from build123d import *

# Parameters (mm, degrees)
T_LE_DE_BASE_PLI_E1_DEPTH = 20
ESQUISSE7_R               = 2
ENL_V_MAT_EXTRU_1_DEPTH   = 25.586228611
ENL_V_MAT_EXTRU_2_DEPTH   = 25.586228611


# Sheet-metal steps are written as plain solids
with BuildPart() as part:
    # Esquisse2 → Tôle de base pliée1 (new body)
    with BuildSketch(Plane.XY):
        with BuildLine():
            Line((-8.571428571, 10.221674877), (-8.571428571, -2.778325123))
            ThreePointArc((-8.571428571, -2.778325123), (-7.985642134, -4.192538686), (-6.571428571, -4.778325123))
            Line((-6.571428571, -4.778325123), (-0.571428571, -4.778325123))
            ThreePointArc((-0.571428571, -4.778325123), (0.842784991, -4.192538686), (1.428571429, -2.778325123))
            Line((1.428571429, -2.778325123), (1.428571429, 10.221674877))
            Line((1.428571429, 10.221674877), (0.428571429, 10.221674877))
            Line((0.428571429, 10.221674877), (0.428571429, -2.778325123))
            ThreePointArc((0.428571429, -2.778325123), (0.13567821, -3.485431904), (-0.571428571, -3.778325123))
            Line((-0.571428571, -3.778325123), (-6.571428571, -3.778325123))
            ThreePointArc((-6.571428571, -3.778325123), (-7.278535353, -3.485431904), (-7.571428571, -2.778325123))
            Line((-7.571428571, -2.778325123), (-7.571428571, 10.221674877))
            Line((-7.571428571, 10.221674877), (-8.571428571, 10.221674877))
        make_face()
    extrude(amount=T_LE_DE_BASE_PLI_E1_DEPTH)

    # Esquisse7 → Enlèv. mat.-Extru.1 (cut, through all)
    with BuildSketch(Plane(origin=(1.428571429, 0, 0), x_dir=(0, 0, -1), z_dir=(1, 0, 0))):
        with Locations(Location((-3, 7.221674877, 0), (0, 0, 180))):
            Circle(ESQUISSE7_R)
        with Locations((-17, 0.221674877)):
            Circle(ESQUISSE7_R)
        with BuildLine():
            Line((-18.341640786, 2.90495645), (-4.341640786, 9.90495645))
            ThreePointArc((-4.341640786, 9.90495645), (-3.689258762, 10.141421845), (-3, 10.221674877))
            Line((-3, 10.221674877), (-20, 10.221674877))
            Line((-20, 10.221674877), (-20, 0.221674877))
            ThreePointArc((-20, 0.221674877), (-19.551952425, 1.798868213), (-18.341640786, 2.90495645))
        make_face()
    extrude(amount=-ENL_V_MAT_EXTRU_1_DEPTH, mode=Mode.SUBTRACT)

    # Esquisse9 → Enlèv. mat.-Extru.2 (cut, through all)
    with BuildSketch(Plane(origin=(1.428571429, 0, 0), x_dir=(0, 0, -1), z_dir=(1, 0, 0))):
        with BuildLine():
            Line((-3, 10.221674877), (0, 10.221674877))
            Line((0, 10.221674877), (0, 7.221674877))
            ThreePointArc((0, 7.221674877), (-0.878679656, 9.34299522), (-3, 10.221674877))
        make_face()
    extrude(amount=-ENL_V_MAT_EXTRU_2_DEPTH, mode=Mode.SUBTRACT)


solid = part.part
Could you check a few things on this model? Use its own coordinates, in mm. A direction names the side the tool comes from. Give positions to 0.01 mm unless a question says otherwise; leave off trailing zeros. Loops run counter-clockwise (first coordinate to the right, second up) from the corner with the lowest first, then second, coordinate; pieces in that order, holes last. Notation, with made-up numbers: (49.5, 46) -> (85.5, 46) arc R24 cw to (85.5, 85) -> close; hole circle Ø7 at (30.5, 85.5). An arc over 180 degrees is marked (long way). Answer as CSV lines item,"result". Start each with the question number.
(1) I'm going to push flat-ended pins straight in: pin 1 Ø1.5 at (x, z) = (0, 12.5) entering from +Y; pin 2 Ø5 at (x, z) = (-2.5, 9.5) entering from +Y; pin 3 Ø4 at (x, z) = (-5, 12.5) entering from +Y. Where does each tip first touch, or does it pass through?
(2) If we section it at A-A on y = 1: Write out the boundary of the cut face in (x, z).
(3) I need wall thicknesses on probe 1 along X at (y, z) = (1.75, 10.25); probe 2 along Y at (x, z) = (-3, 4.5); probe 3 along Y at (x, z) = (-8.05, 17). Which ranges of each line are inside material? Lowest first, please.
(4) Which directions (+Z, -Z, +X, -X, +Y, -Y) give clear straight access to the entire face, cutting with the end or side of a thin tool? Please do faces 1 (the cylindrical face through (-7.271, -3.493, 9.86)), 2 (the cylindrical face through (-8.1, 0.3, 19)).
(5) If we section it at B-B on z = 3.5: Write out the boundary of the cut face in (x, y), then the cut area to 3 significant figures.
(6) If we section it at D-D on y = 9.5: Write out the boundary of the cut face in (x, z).
(7) We'd pull the mould along X, two halves only. Please class faces 3 (the flat face through (-8.571, 2, 8)), 4 (the flat face through (0.429, 2, 8)), 5 (the flat face through (-4, -4.778, 10)): released by +X, released by -X, zero draft, split by the parting line, or undercut.
(8) If we section it at C-C on x = 0.75: Write out the boundary of the cut face in (y, z), then the cut area to 3 significant figures.
Computed:
1,pin 1,"stops at y = 6.13"
1,pin 2,"stops at y = -3.6"
1,pin 3,"stops at y = -3.68"
2,outline,"(-8.57, 0) -> (-7.57, 0) -> (-7.57, 15.16) -> (-8.57, 15.16) -> close; (-8.57, 18.84) -> (-7.57, 18.84) -> (-7.57, 19.9) -> (-8.57, 19.9) -> close; (0.43, 0) -> (1.43, 0) -> (1.43, 15.16) -> (0.43, 15.16) -> close; (0.43, 18.84) -> (1.43, 18.84) -> (1.43, 19.9) -> (0.43, 19.9) -> close"
3,probe 1,"x = -8.57 to -7.57, 0.43 to 1.43"
3,probe 2,"y = -4.78 to -3.78"
3,probe 3,"y = -4.13 to -1.78, 2.22 to 3.58"
4,face 1,"+Z, -Z, +Y"
4,face 2,"+X, -X"
5,outline,"(-8.57, -2.78) arc R2 ccw to (-6.57, -4.78) -> (-0.57, -4.78) arc R2 ccw to (1.43, -2.78) -> (1.43, 5.29) -> (0.43, 5.29) -> (0.43, -2.78) arc R1 cw to (-0.57, -3.78) -> (-6.57, -3.78) arc R1 cw to (-7.57, -2.78) -> (-7.57, 5.29) -> (-8.57, 5.29) -> close; (-8.57, 9.16) -> (-7.57, 9.16) -> (-7.57, 10.18) -> (-8.57, 10.18) -> close; (0.43, 9.16) -> (1.43, 9.16) -> (1.43, 10.18) -> (0.43, 10.18) -> close"
5,area,"28.9 mm2"
6,outline,"(-8.57, 1.05) -> (-7.57, 1.05) -> (-7.57, 5.15) -> (-8.57, 5.15) -> close; (0.43, 1.05) -> (1.43, 1.05) -> (1.43, 5.15) -> (0.43, 5.15) -> close"
7,face 3,"released by -X"
7,face 4,"undercut"
7,face 5,"zero draft"
8,outline,"(-4.28, 0) -> (7.22, 0) arc R3 ccw to (9.9, 4.34) -> (2.9, 18.34) arc R3 ccw to (0.22, 20) -> (-4.28, 20) -> close; hole circle Ø4 at (0.22, 17); hole circle Ø4 at (7.22, 3)"
8,area,"196 mm2"
